Part model, mm, in its own coordinate system. Face numbers are marked on the shaded views. A direction names the side the tool comes from. Coordinates: 2 decimals unless noted, no trailing zeros. Loops run counter-clockwise (first coordinate to the right, second up) from the corner with the lowest first, then second, coordinate; pieces in that order, holes last. Notation, with made-up numbers: (30, 35) -> (86, 35) arc R29 cw to (86, 62) -> close; hole circle Ø11 at (64, 0). An arc over 180 degrees is marked (long way). One line per question, with ' | ' between items. Start each with the question number.
1) Drop flat-ended pins along their axis: pin 1 (4 mm diameter, centred on y = 19.5, z = 10.5, fed in from -X); pin 2 (0.8 mm diameter, centred on x = 4, y = 17, fed in from +Z); pin 3 (8 mm diameter, centred on y = -5, z = 10.5, fed in from -X). Give the stop position or say it passes through.
2) Two-plate mould, pull along X, no slides. Class the marked faces 1, 2 and 3: released by +X, released by -X, zero draft, split by the parting line, or undercut.
3) Probe L1, parallel to Y at x = 29, z = 1.05; L2, parallel to Y at x = -5, z = 19; L3, parallel to Y at x = -22.5, z = 10.5. List the from-to ranges inside material, lowest first. Write a range as from..to.
4) Cut at B-B (x = 25.5). List the corners of the cut face in (y, z), plus the area to 3 significant figures.
5) Cut at C-C (y = 21). Count the separate pieces of the cut face and the enclosed holes in it, plus the area to 3 significant figures.
6) 3-axis set-ups, long thin cutter, end or side, ignore diameter. For the marked faces 4, 5, 6, 7 and 8: which of +Z, -Z, +X, -X, +Y, -Y reach the whole face in a straight line?
7) Cut at A-A (x = -29). List the corners of the cut face in (y, z).
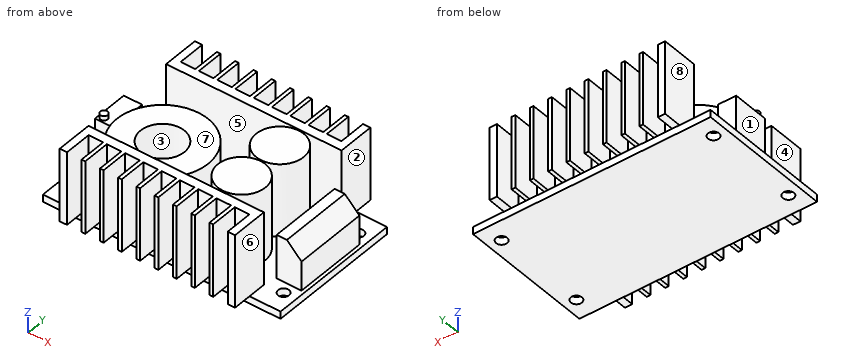
from build123d import *

# Parameters (mm, degrees)
SKETCH_1_W          = 65
SKETCH_1_H          = 37
EXTRUDE_1_DEPTH     = 2
EXTRUDE_2_DEPTH     = 20
SKETCH_3_R          = 6.5
EXTRUDE_3_DEPTH     = 20
SKETCH_4_R          = 12.5
SKETCH_4_R_2        = 6
EXTRUDE_4_DEPTH     = 12
SKETCH_5_W          = 5
SKETCH_5_H          = 10
EXTRUDE_5_DEPTH     = 10
SKETCH_6_R          = 1
EXTRUDE_6_DEPTH     = 1.2
SKETCH_7_W          = 6.798722996
SKETCH_7_H          = 20.12306807
EXTRUDE_7_DEPTH     = 12
CHAMFER_1_SIZE      = 4
SKETCH_8_R          = 1.5
CUT_EXTRUDE_1_DEPTH = 3


with BuildPart() as part:
    # Эскиз1 → Бобышка-Вытянуть1 (new body)
    with BuildSketch(Plane.XY):
        Rectangle(SKETCH_1_W, SKETCH_1_H)
    extrude(amount=EXTRUDE_1_DEPTH)

    # Эскиз2 → Бобышка-Вытянуть2 (add)
    with BuildSketch(Plane.XY.offset(2)):
        Polygon((-24, 23.5), (-24, 13.5), (24, 13.5), (24, 23.5), (22, 23.5), (22, 16), (18, 16), (18, 23.5), (17, 23.5), (17, 16), (13, 16), (13, 23.5), (12, 23.5), (12, 16), (8, 16), (8, 23.5), (7, 23.5), (7, 16), (3, 16), (3, 23.5), (2, 23.5), (2, 16), (-2, 16), (-2, 23.5), (-3, 23.5), (-3, 16), (-7, 16), (-7, 23.5), (-8, 23.5), (-8, 16), (-12, 16), (-12, 23.5), (-13, 23.5), (-13, 16), (-17, 16), (-17, 23.5), (-18, 23.5), (-18, 16), (-22, 16), (-22, 23.5), align=None)
        Polygon((22, -23.5), (24, -23.5), (24, -13.5), (-24, -13.5), (-24, -23.5), (-22, -23.5), (-22, -16), (-18, -16), (-18, -23.5), (-17, -23.5), (-17, -16), (-13, -16), (-13, -23.5), (-12, -23.5), (-12, -16), (-8, -16), (-8, -23.5), (-7, -23.5), (-7, -16), (-3, -16), (-3, -23.5), (-2, -23.5), (-2, -16), (2, -16), (2, -23.5), (3, -23.5), (3, -16), (7, -16), (7, -23.5), (8, -23.5), (8, -16), (12, -16), (12, -23.5), (13, -23.5), (13, -16), (17, -16), (17, -23.5), (18, -23.5), (18, -16), (22, -16), align=None)
    extrude(amount=EXTRUDE_2_DEPTH)

    # Эскиз3 → Бобышка-Вытянуть3 (add)
    with BuildSketch(Plane.XY.offset(2)):
        with Locations((12.5, 6.691570058)):
            Circle(SKETCH_3_R)
        with Locations((12.5, -6.612413993)):
            Circle(SKETCH_3_R)
    extrude(amount=EXTRUDE_3_DEPTH)

    # Эскиз4 → Бобышка-Вытянуть4 (add)
    with BuildSketch(Plane.XY.offset(2)):
        with Locations((-14.373526478, 0)):
            Circle(SKETCH_4_R)
        with Locations((-14.373526478, 0)):
            Circle(SKETCH_4_R_2, mode=Mode.SUBTRACT)
    extrude(amount=EXTRUDE_4_DEPTH)

    # Эскиз5 → Бобышка-Вытянуть5 (add)
    with BuildSketch(Plane.XY.offset(2)):
        with Locations((-29.649429854, 4.142703247)):
            Rectangle(SKETCH_5_W, SKETCH_5_H)
    extrude(amount=EXTRUDE_5_DEPTH)

    # Эскиз6 → Бобышка-Вытянуть6 (add)
    with BuildSketch(Plane.XY.offset(12)):
        with Locations((-30.813495229, 0.582032688)):
            Circle(SKETCH_6_R)
    extrude(amount=EXTRUDE_6_DEPTH)

    # Эскиз7 → Бобышка-Вытянуть7 (add)
    with BuildSketch(Plane.XY.offset(2)):
        with Locations((28.195350692, 0)):
            Rectangle(SKETCH_7_W, SKETCH_7_H)
    extrude(amount=EXTRUDE_7_DEPTH)

    # Фаска1
    chamfer_1_edges = [part.edges().sort_by_distance(p)[0] for p in [
        (31.59471219, 0, 14),
    ]]
    chamfer(chamfer_1_edges, length=CHAMFER_1_SIZE)

    # Эскиз8 → Вырез-Вытянуть1 (cut, through all)
    with BuildSketch(Plane.XY.offset(2)):
        with Locations((-29, 13)):
            Circle(SKETCH_8_R)
        with Locations((29, 13)):
            Circle(SKETCH_8_R)
        with Locations((29, -13)):
            Circle(SKETCH_8_R)
        with Locations((-29, -13)):
            Circle(SKETCH_8_R)
    extrude(amount=-CUT_EXTRUDE_1_DEPTH, mode=Mode.SUBTRACT)


solid = part.part
Reported:
1) pin 1: stops at x = -24 | pin 2: stops at z = 2 | pin 3: stops at x = -26.83
2) face 1: released by -X | face 2: released by +X | face 3: undercut
3) L1: y = -18.5..-14.5, -11.5..11.5, 14.5..18.5 | L2: y = -16..-13.5, 13.5..16 | L3: y = -23.5..-13.5, -9.5..9.5, 13.5..23.5
4) outline: (-18.5, 0) -> (18.5, 0) -> (18.5, 2) -> (10.06, 2) -> (10.06, 14) -> (-10.06, 14) -> (-10.06, 2) -> (-18.5, 2) -> close | area: 315 mm²
5) separate pieces: 10 | enclosed holes: 0 | area: 240 mm²
6) face 4: +Z, -X, -Y | face 5: +Z, +X, -X | face 6: +Z, +X, +Y, -Y | face 7: +Z, -X | face 8: +Z, -X, +Y
7) outline: (-18.5, 0) -> (-14.5, 0) -> (-14.5, 2) -> (-18.5, 2) -> close; (-11.5, 0) -> (11.5, 0) -> (11.5, 2) -> (9.14, 2) -> (9.14, 12) -> (-0.86, 12) -> (-0.86, 2) -> (-11.5, 2) -> close; (14.5, 0) -> (18.5, 0) -> (18.5, 2) -> (14.5, 2) -> close
